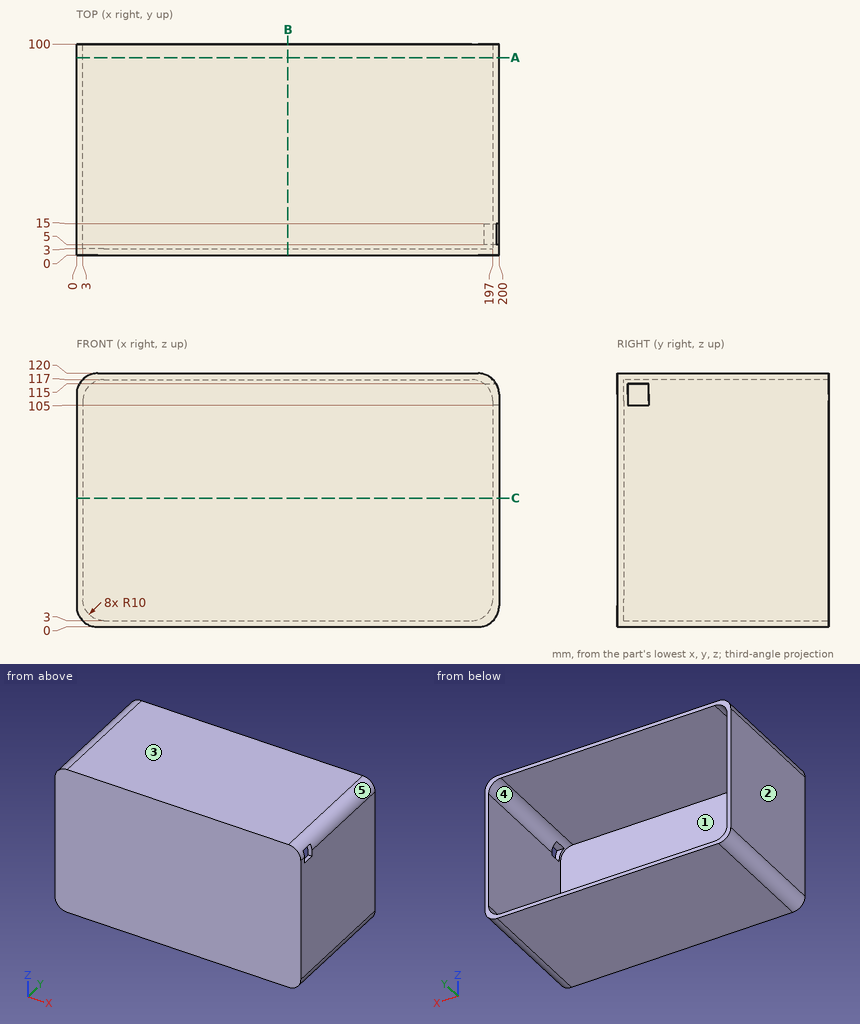
Study the drawing (mm; zero at the part's minimum x, y, z) and answer. A direction names the side the tool comes from. Give positions to 0.01 mm unless a question says otherwise; leave off trailing zeros. Loops run counter-clockwise (first coordinate to the right, second up) from the corner with the lowest first, then second, coordinate; pieces in that order, holes last. Notation, with made-up numbers: M -18.5,56 L 1.5,56 A25 ccw 1.5,91 Z; hole C 55,-5.75 d5. An arc over 180 degrees is marked long. One line per item, written item: value. Start each with the question number.
1. Find the intervals of material crossed by probe 1 along X at (y, z) = (7, 24.5); probe 2 along Z at (x, y) = (171, 37.5); probe 3 along Y at (x, z) = (132, 62), in increasing order.
2. Which of the six approach directions +Z, -Z, +X, -X, +Y, -Y give full straight-line access (tool end or side, diameter ignored) to the marked faces 4 and 5?
3. Find section C-C (z = 61). Give the vertices of the cut face in (x, y).
4. Find section A-A (y = 93.5). Give the vertices of the cut face in (x, z).
5. Each of these flat-tipped pins is pushed along its axis until it touches: P1, Ø3.5, axis at x = 195, z = 111, coming from the -Y side; P2, Ø1.5, axis at x = 150, z = 46, coming from the +Y side; P3, Ø1.5, axis at x = 198, y = 11.5, coming from the +Z side; P4, Ø1.7, axis at x = 197, y = 8, coming from the -Z side. Where does it stop, or does it pass through?
6. Determine the mould class of the marked faces 1, 2 and 3 for opening direction Z: released by +Z, released by -Z, zero draft, split by the parting line, or undercut.
7. Find section B-B (x = 100). Give the vertices of the cut face in (y, z).
Reported:
1. probe 1: x = 0 to 3, 197 to 200
1. probe 2: z = 0 to 3, 117 to 120
1. probe 3: y = 0 to 3
2. face 4: +Y
2. face 5: +Z, +X, +Y, -Y
3. outline: M 0,0 L 200,0 L 200,100 L 197,100 L 197,3 L 3,3 L 3,100 L 0,100 Z
4. outline: M 0,10 A10 ccw 10,0 L 190,0 A10 ccw 200,10 L 200,110 A10 ccw 190,120 L 10,120 A10 ccw 0,110 Z; hole M 3,13 A10 ccw 13,3 L 187,3 A10 ccw 197,13 L 197,107 A10 ccw 187,117 L 13,117 A10 ccw 3,107 Z
5. P1: stops at y = 0
5. P2: stops at y = 3
5. P3: stops at z = 116.89
5. P4: stops at z = 2.11
6. face 1: undercut
6. face 2: zero draft
6. face 3: released by +Z
7. outline: M 0,0 L 100,0 L 100,3 L 3,3 L 3,117 L 100,117 L 100,120 L 0,120 Z
